Could you check a few things on this drawing? It's one solid part, dimensions in mm from its lowest x, y, z. A direction names the side the tool comes from. Give positions to 0.01 mm unless a question says otherwise; leave off trailing zeros. Order: outer loops, then holes, each group sorted by start corner. A loop starts at its lowest first (then second) coordinate and runs counter-clockwise, first axis right, second up. Notation, with made-up numbers: (8.25, 4) -> (15.25, 4) arc R17 ccw to (15.25, 18) -> close; hole circle Ø6 at (-15, 40). An arc over 180 degrees is marked (long way). Write each question's results on one line, items separated by ' | '. Start each with the question number.
Q1. Imagine slicing it at D-D, the plane y = 31.5. Please give me the cut outline in (x, z), then the cut area to 3 significant figures.
Q2. Thinking about a two-plate mould opening in X: for the marked faces 1, 2 and 3, which applies, pulls with the +X half, pulls with the -X half, needs draft (parallel to the pull), parting line crosses it, or undercut?
Q3. Imagine slicing it at C-C, the plane z = 5.25. Please give me the cut outline in (x, y).
Q4. I'm going to push flat-ended pins straight in: pin 1 (5.5 mm diameter, centred on x = 2, y = 3.5, fed in from +Z); pin 2 (10 mm diameter, centred on x = 26, y = 22.5, fed in from +Z); pin 3 (1.5 mm diameter, centred on x = 3, z = 5, fed in from -Y); pin 4 (1.5 mm diameter, centred on y = 3.5, z = 4.5, fed in from -X). Where does each tip first touch, or does it pass through?
Q5. For the marked faces 4, 5, 6, 7 and 8, which set-ups out of +Z, -Z, +X, -X, +Y, -Y let a thin tool reach every point of the face, with its end or its side?
Q6. Imagine slicing it at B-B, the plane y = 17.5. Please give me the cut outline in (x, z).
Q7. I need wall thicknesses on line 1 along Y through (x, z) = (2.5, 0.5); line 2 along X through (y, z) = (3.5, 6.25); line 3 along Y through (x, z) = (32.5, 0.7). Which ranges of each line are inside material? Lowest first, please. Write a range as [from, to].
Q8. Imagine slicing it at A-A, the plane x = 3.5. Please give me the cut outline in (y, z).
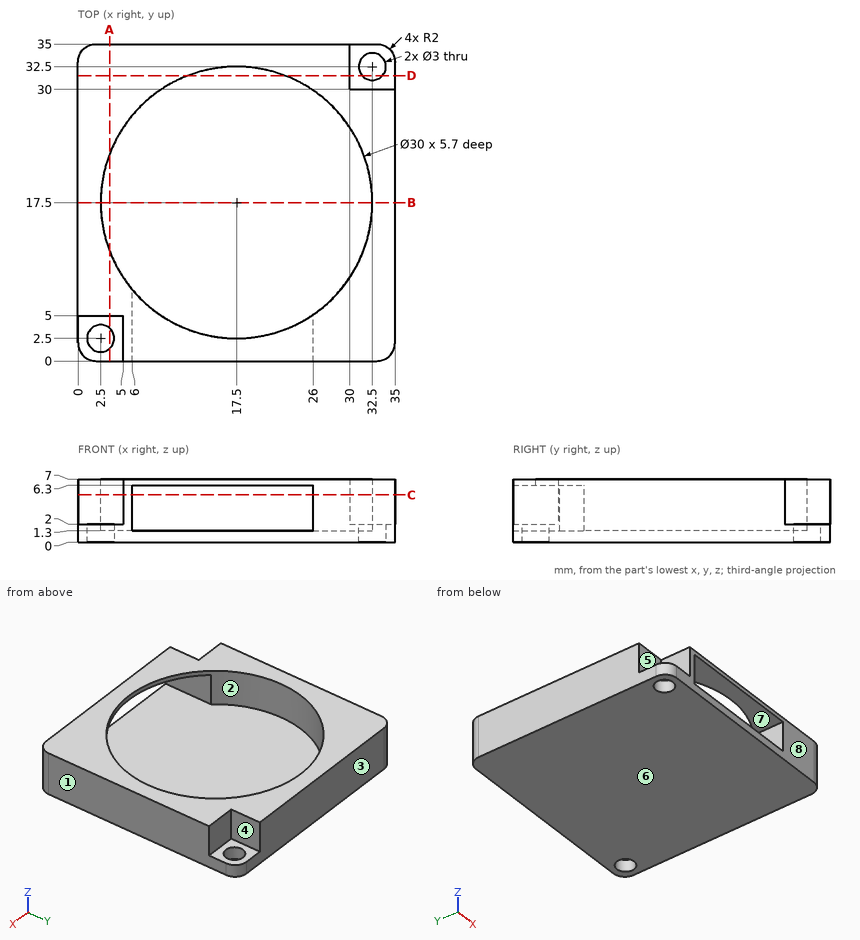
Geometry check:
1) outline: (0, 0) -> (31.38, 0) -> (31.38, 2) -> (30, 2) -> (30, 7) -> (22.89, 7) -> (22.89, 1.3) -> (12.11, 1.3) -> (12.11, 7) -> (0, 7) -> close; (33.62, 0) -> (35, 0) -> (35, 2) -> (33.62, 2) -> close | area: 154 mm²
2) face 1: pulls with the +X half | face 2: undercut | face 3: needs draft
3) outline: (0, 5) -> (5, 5) -> (5, 0) -> (6, 0) -> (6, 7.87) arc R15 cw (long way) to (26, 5.14) -> (26, 0) -> (33, 0) arc R2 ccw to (35, 2) -> (35, 30) -> (30, 30) -> (30, 35) -> (2, 35) arc R2 ccw to (0, 33) -> close
4) pin 1: z = 7 | pin 2: z = 1.3 | pin 3: y = 5 | pin 4: x = 5
5) face 4: +Z, +X, +Y | face 5: +Z, -X, -Y | face 6: -Z, +X, -X, +Y, -Y | face 7: -Y | face 8: +Z, -Z, +X, -X, -Y
6) outline: (0, 0) -> (35, 0) -> (35, 7) -> (32.5, 7) -> (32.5, 1.3) -> (2.5, 1.3) -> (2.5, 7) -> (0, 7) -> close
7) line 1: [0, 1], [4, 35] | line 2: [5, 6], [26, 35] | line 3: [0, 31], [34, 35]
8) outline: (0, 0) -> (1.38, 0) -> (1.38, 2) -> (0, 2) -> close; (3.62, 0) -> (35, 0) -> (35, 7) -> (22.89, 7) -> (22.89, 1.3) -> (12.11, 1.3) -> (12.11, 7) -> (5, 7) -> (5, 2) -> (3.62, 2) -> close
